Geometry: final body of the model. Coordinates: model frame, mm. Face numbers are marked on the shaded views. Round coordinates to 2 decimals unless told otherwise and drop trailing zeros. Write each loop counter-clockwise with the first axis right and the second up, starting at its lowest first coordinate (ties: lowest second). Pieces come first, ordered by that corner, then holes. Notation, with made-up numbers: M -32,-8 L -5,-8 A23 cw -5,25 Z; hole C 62,-1 d4. An arc over 180 degrees is marked long. Use one line per item in the form item = value. Start each with the question number.
Autodesk Inventor part; units mm, degrees
ref_plane "Start Plane" through (0, 0, -4.9897) normal (0, 0, 1) x (1, 0, 0)
ref_plane "End Plane" through (0, 0, 105.0166) normal (0, 0, 1) x (1, 0, 0)
ref_plane "Work Plane4" through (-9.4897, -4.8737, -6.8509) normal (0.4807, 0.2469, -0.8414) x (-0.4571, -0.7483, -0.4807)
ref_plane "Start Plane" through (0, 0, -4.9897) normal (0, 0, 1) x (1, 0, 0)
ref_plane "End Plane" through (0, 0, 105.0166) normal (0, 0, 1) x (1, 0, 0)
sketch "Sketch" plane through (0, 0, 0) normal (0, 0, 1) x (1, 0, 0)
  circle A0 centre (0, 0) radius 6.9342
  circle A1 centre (0, 0) radius 10.668
  dimension "d0" = 21.336
  dimension "d1" = 3.7338
extrude "Body" add sketch "Sketch" along normal up to surface (110.0063 mm away) from surface at -4.9897
sketch "Sketch3" plane through (0, 0, 0) normal (0, 0, 1) x (1, 0, 0)
  line L0 (0, 0) -> (10, 0)
ref_plane "Work Plane3" through (0, 0, 0) normal (0, -1, 0) x (1, 0, 0)
sketch "Sketch4" plane through (0, 0, 0) normal (0, -1, 0) x (1, 0, 0)
  line L0 (-2, -4.9897) -> (12, -4.9897)
  line L1 (-2, 105.0166) -> (12, 105.0166)
  dimension "d7" = 110.0063
ref_plane "Work Plane4" through (-9.4897, -4.8737, -6.8509) normal (0.4807, 0.2469, -0.8414) x (-0.4571, -0.7483, -0.4807)
split "Split1" plane through (-9.4897, -4.8737, -6.8509) removes the side toward (0.4807, 0.2469, -0.8414)
ref_plane "Work Plane5" through (6.4449, -8.5011, -9.0952) normal (-0.392, 0.517, -0.761) x (0.3573, 0.8478, 0.392)
split "Split2" plane through (6.4449, -8.5011, -9.0952) removes the side toward (-0.392, 0.517, -0.761)
ref_plane "Work Plane6" through (-10.5607, -1.5089, 115.9586) normal (0.7772, 0.111, 0.6194) x (0.627, -0.0533, -0.7772)
split "Split3" plane through (-10.5607, -1.5089, 115.9586) removes the side toward (0.7772, 0.111, 0.6194)
ref_plane "Work Plane7" through (0, -10.668, 105.0198) normal (0, 0.2353, 0.9719) x (1, 0, 0)
split "Split4" plane through (0, -10.668, 105.0198) removes the side toward (0, 0.2353, 0.9719)
ref_plane "Work Plane8" through (8.1097, -2.9756, 133.7039) normal (0.1452, -0.9053, 0.3992) x (0.0697, 0.4118, 0.9086)
sketch "Sketch5" plane through (8.1097, -2.9756, 133.7039) normal (0.1452, -0.9053, 0.3992) x (0.0697, 0.4118, 0.9086)
  circle A0 centre (-39.4415, 1.4606) radius 3
  point P0 (-120.8228, -8.7403)
hole "Hole1" at (3.9184, -19.3703, 98.047) direction (-0.1452, 0.9053, -0.3992) diameter 5.4 depth 20 tip angle 118
equation "\"d0\" = G_H"
equation "\"d1\" = G_T"
equation "\"d2\" = G_L"
equation "\"G_H\" = 21.336"
equation "\"G_T\" = 3.7338"
equation "\"G_L\" = 110.00626"
equation "\"G_OFFSET_START\" = 4.98966"
equation "\"G_OFFSET_END\" = 2.57893"
equation "\"d4\" = -G_OFFSET_START"
equation "\"d5\" = G_OFFSET_END + B_L"
equation "\"B_L\" = 102.43767"
properties part number "ANSI - 1/2 x 0.147 - 4.331" material "Steel, Mild"
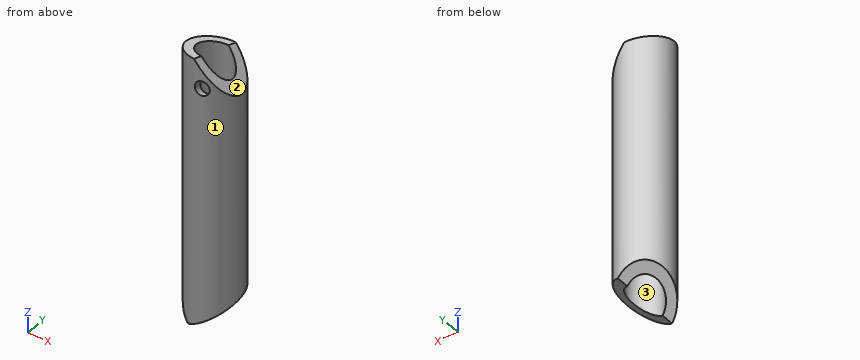
1. Section query C-C (y = 4.25). Return loops of the section in (x, z), then the cut area to 3 significant figures.
2. Pull-direction query (X, two-part tool) for the marked faces 1, 2 and 3; classes: released by +X, released by -X, zero draft, split by the parting line, or undercut.
3. Ray query, probe 1 along Y at (x, z) = (0, 77); probe 2 along X at (y, z) = (-0.5, 10.5); probe 3 along X at (y, z) = (-1.5, 41). Return the intervals inside material, ascending.
4. Contact query for flat-ended pins moving along their axis: pin 1 (12 mm diameter, centred on x = 4, y = 6.5, fed in from +Z); pin 2 (5 mm diameter, centred on y = -4.5, z = 80.5, fed in from +X); pin 3 (4 mm diameter, centred on x = 0.5, y = -4.5, fed in from -Z); pin 4 (8 mm diameter, centred on y = 3.5, z = 71, fed in from +X). Output: stop coordinate, or through.
5. Section query B-B (z = 81). Return loops of the section in (x, y), then the cut area to 3 significant figures.
6. Section query A-A (y = 0). Return loops of the section in (x, z), then the cut area to 3 significant figures.
Checks:
q1.outline = M -9.78,7.93 L -5.48,5.71 L -5.48,101.41 L -9.78,101.41 Z; M 5.48,4.38 L 9.78,6.84 L 9.78,89.4 L 5.48,94.8 Z
q1.area = 780 mm^2
q2.face_1 = split by the parting line
q2.face_2 = released by +X
q2.face_3 = undercut
q3.probe_1 = -10.67 to -6.93, 6.93 to 10.67
q3.probe_2 = -10.66 to -6.92, 6.92 to 10.66
q3.probe_3 = -10.56 to -6.77, 6.77 to 10.56
q4.pin_1 = 100.83
q4.pin_2 = 10.48
q4.pin_3 = through
q4.pin_4 = 10.67
q5.outline = C 0,0 d21.34; hole C 0,0 d13.87
q5.area = 206 mm^2
q6.outline = M -10.67,5.5 L -6.93,3.57 L -6.93,102.44 L -10.67,102.44 Z; M 6.93,3.96 L 10.67,6.1 L 10.67,89.05 L 6.93,93.74 Z
q6.area = 688 mm^2
